from build123d import *

# Parameters (mm, degrees)
TUBE_R        = 23.75
TUBE_R_2      = 23
TUBE_DEPTH    = 6
SKETCH004_R   = 1
PAD002_DEPTH  = 1
SKETCH006_R   = 16.6
SKETCH006_R_2 = 16.3
PAD003_DEPTH  = 2


with BuildPart() as tube:
    # Tube → Tube (new body)
    with BuildSketch(Plane.XY):
        Circle(TUBE_R)
        Circle(TUBE_R_2, mode=Mode.SUBTRACT)
    extrude(amount=TUBE_DEPTH)


with BuildPart() as fusion002:
    # Sketch004 → Pad002 (new body)
    with BuildSketch(Plane.XY):
        with BuildLine():
            ThreePointArc((32, 0), (0, 32), (-32, 0))
            Line((-32, 0), (-32, -30.055735))
            ThreePointArc((-32, -30.055735), (-30.551858, -33.551858), (-27.055735, -35))
            Line((-27.055735, -35), (26.427752, -35))
            ThreePointArc((26.427752, -35), (30.367926, -33.367926), (32, -29.427752))
            Line((32, -29.427752), (32, 0))
        make_face()
        with Locations((-27, -25)):
            Circle(SKETCH004_R, mode=Mode.SUBTRACT)
        with Locations((27, -25)):
            Circle(SKETCH004_R, mode=Mode.SUBTRACT)
        with Locations((24, 14)):
            Circle(SKETCH004_R, mode=Mode.SUBTRACT)
        with Locations((-24, 14)):
            Circle(SKETCH004_R, mode=Mode.SUBTRACT)
        with BuildLine():
            ThreePointArc((-6, 16), (-9, 13), (-6, 10))
            Line((-6, 10), (6, 10))
            ThreePointArc((6, 10), (9, 13), (6, 16))
            Line((6, 16), (-6, 16))
        make_face(mode=Mode.SUBTRACT)
    extrude(amount=PAD002_DEPTH)

    # Sketch006 → Pad003 (join)
    with BuildSketch(Plane.XY):
        Circle(SKETCH006_R)
        Circle(SKETCH006_R_2, mode=Mode.SUBTRACT)
    extrude(amount=PAD003_DEPTH)

    # Fusion002: union Tube
    add(tube.part)


solid = fusion002.part
Can you work these out from the model? Positions are in its coordinate system, mm. A direction names the side the tool comes from. Give positions to 0.01 mm unless a question says otherwise; leave off trailing zeros. Order: outer loops, then holes, each group sorted by start corner. A loop starts at its lowest first (then second) coordinate and runs counter-clockwise, first axis right, second up. Notation, with made-up numbers: M 51,89 L 83,89 A31 ccw 83,115 Z; hole C 43.5,71 d8. An arc over 180 degrees is marked long. Use a Markdown table: item, result. Add a question column.
Item 1: Will these pins go through, and if not, where does the flat tip stop? pin 1 (8 mm diameter, centred on x = 7, y = 24.5, fed in from +Z); pin 2 (15 mm diameter, centred on x = 7, y = 4, fed in from +Z); pin 3 (2 mm diameter, centred on x = 21.5, z = 3.5, fed in from -Y); pin 4 (1.5 mm diameter, centred on x = 12, z = 3, fed in from -Y).
Item 2: Suppose I cut it at C-C (z = 3.65). List the corners of the cut face in (x, y) for me.
Item 3: Suppose I cut it at D-D (y = 1.5). List the corners of the cut face in (x, z) for me, then the cut area to 3 significant figures.
Item 4: If I drill on L1, parallel to Y at x = 0, z = 4.5; L2, parallel to X at y = 7, z = 2.6; L3, parallel to Y at x = -18.5, z = 2.85, over which ranges is the centre line in solid material (lowest first)? Write a range as [from, to].
Item 5: Suppose I cut it at A-A (y = -25). List the corners of the cut face in (x, z) for me.
Item 6: We'd pull the mould along X, two halves only. Please class faces 4 (the cylindrical face through (-5.149, -23.185, 3.465)), 5 (the flat face through (7, -23, 1)), 6 (the flat face through (0, -1, 1)): +X half, -X half, draft (parallel to the pull), parting line (faces both ways), or undercut.
Item 7: Suppose I cut it at B-B (x = 7). List the corners of the cut face in (y, z) for me, then the cut area to 3 significant figures.
Item 8: For faces 1 (the cylindrical face through (0.704, 31.992, 0.493)), 2 (the cylindrical face through (-2.994, 22.804, 3.465)), 3 (the cylindrical face through (-8.36, 11.15, 0.49)), which set-ups out of +Z, -Z, +X, -X, +Y, -Y let a thin tool reach every point of the face, with its end or its side?
Answer sheet:
| question | item | result |
|---|---|---|
| 1 | pin 1 | stops at z = 6 |
| 1 | pin 2 | stops at z = 1 |
| 1 | pin 3 | stops at y = -11.99 |
| 1 | pin 4 | stops at y = -20.92 |
| 2 | outline | C 0,0 d47.5; hole C 0,0 d46 |
| 3 | outline | M -31.96,0 L 31.96,0 L 31.96,1 L 23.7,1 L 23.7,6 L 22.95,6 L 22.95,1 L 16.53,1 L 16.53,2 L 16.23,2 L 16.23,1 L -16.23,1 L -16.23,2 L -16.53,2 L -16.53,1 L -22.95,1 L -22.95,6 L -23.7,6 L -23.7,1 L -31.96,1 Z |
| 3 | area | 72.0 mm² |
| 4 | L1 | y = [-23.75, -23], [23, 23.75] |
| 4 | L2 | x = [-22.69, -21.91], [21.91, 22.69] |
| 4 | L3 | y = [-14.89, -13.67], [13.67, 14.89] |
| 5 | outline | M -32,0 L -28,0 L -28,1 L -32,1 Z; M -26,0 L 26,0 L 26,1 L -26,1 Z; M 28,0 L 32,0 L 32,1 L 28,1 Z |
| 6 | face 4 | parting line |
| 6 | face 5 | draft |
| 6 | face 6 | undercut |
| 7 | outline | M -35,0 L 10.17,0 L 10.17,1 L -14.72,1 L -14.72,2 L -15.05,2 L -15.05,1 L -21.91,1 L -21.91,6 L -22.69,6 L -22.69,1 L -35,1 Z; M 14.72,0 L 15.05,0 L 15.05,2 L 14.72,2 Z; M 15.83,0 L 31.22,0 L 31.22,1 L 22.69,1 L 22.69,6 L 21.91,6 L 21.91,1 L 15.83,1 Z |
| 7 | area | 69.4 mm² |
| 8 | face 1 | +Z, -Z, +Y |
| 8 | face 2 | +Z |
| 8 | face 3 | +Z, -Z |
